from build123d import *

# Parameters (mm, degrees)
SKETCH_1_R          = 11
EXTRUDE_1_DEPTH     = 3.5
SKETCH_2_R          = 5
EXTRUDE_2_DEPTH     = 11.5
SKETCH_3_R          = 4
CUT_EXTRUDE_1_DEPTH = 22.610182785
SKETCH_4_R          = 1.75
CUT_EXTRUDE_2_DEPTH = 20.345542122


with BuildPart() as part:
    # 草图1 → 凸台-拉伸1 (new body)
    with BuildSketch(Plane(origin=(0, 0, 0), x_dir=(1, 0, 0), z_dir=(0, 1, 0))):
        with Locations(Location((0, 0, 0), (0, 0, 270))):
            Circle(SKETCH_1_R)
    extrude(amount=EXTRUDE_1_DEPTH)

    # 草图2 → 凸台-拉伸2 (add)
    with BuildSketch(Plane(origin=(0, 3.5, 0), x_dir=(1, 0, 0), z_dir=(0, 1, 0))):
        with Locations(Location((0, 0, 0), (0, 0, 270))):
            Circle(SKETCH_2_R)
    extrude(amount=EXTRUDE_2_DEPTH)

    # 草图3 → 切除-拉伸1 (cut, through all)
    with BuildSketch(Plane(origin=(0, 15, 0), x_dir=(1, 0, 0), z_dir=(0, 1, 0))):
        with Locations(Location((0, 0, 0), (0, 0, 270))):
            Circle(SKETCH_3_R)
    extrude(amount=-CUT_EXTRUDE_1_DEPTH, mode=Mode.SUBTRACT)

    # 草图4 → 切除-拉伸2 (cut, through all)
    with BuildSketch(Plane(origin=(0, 3.5, 0), x_dir=(1, 0, 0), z_dir=(0, 1, 0))):
        with Locations(Location((0, 8, 0), (0, 0, 270))):
            Circle(SKETCH_4_R)
        with Locations(Location((8, 0, 0), (0, 0, 270))):
            Circle(SKETCH_4_R)
        with Locations(Location((0, -8, 0), (0, 0, 270))):
            Circle(SKETCH_4_R)
        with Locations(Location((-8, 0, 0), (0, 0, 270))):
            Circle(SKETCH_4_R)
    extrude(amount=-CUT_EXTRUDE_2_DEPTH, mode=Mode.SUBTRACT)


solid = part.part
The model under review builds one solid part; all positions refer to its coordinate system, in mm. A direction names the side the tool comes from. Round coordinates to 2 decimals unless told otherwise and drop trailing zeros. Loops run counter-clockwise (first coordinate to the right, second up) from the corner with the lowest first, then second, coordinate; pieces in that order, holes last. Notation, with made-up numbers: (-12, 7.5) -> (43, 7.5) arc R35 ccw to (43, 43.5) -> close; hole circle Ø6 at (55, -35). An arc over 180 degrees is marked (long way). Return JSON: item names as keys, results as strings.
(1) Add section C-C on x = 7. Write out the cut boundary in (y, z), plus the area to 3 significant figures.
Solved:
{"outline": "(0, -8.49) -> (3.5, -8.49) -> (3.5, -1.44) -> (0, -1.44) -> close; (0, 1.44) -> (3.5, 1.44) -> (3.5, 8.49) -> (0, 8.49) -> close", "area": "49.3 mm2"}
(2) The part is to be moulded in two halves that separate along Z. For faces 3 (the cylindrical face through (-3.905, 7.605, -0.867)), 4 (the cylindrical face through (-10.74, 1.73, -2.38)), 5 (the cylindrical face through (0.526, 1.774, 9.669)), 6 (the flat face through (-5, 3.5, 2)), say which applies: released by +Z, released by -Z, zero draft, split by the parting line, or undercut.
Solved:
{"face 3": "undercut", "face 4": "split by the parting line", "face 5": "undercut", "face 6": "zero draft"}
(3) For faces 1 (the cylindrical face through (-4.88, 9.17, -1.08)), 2 (the cylindrical face through (-9.55, 1.77, 0.81)), list the 3-axis set-ups (+Z, -Z, +X, -X, +Y, -Y) from which the entire face can be reached by the end or side of a thin tool; tool diameter is ignored.
Solved:
{"face 1": "+Y", "face 2": "+Y, -Y"}
(4) Add section D-D on y = 10.5. Write out the cut boundary in (x, z), plus the area to 3 significant figures.
Solved:
{"outline": "circle Ø10 at (0, 0); hole circle Ø8 at (0, 0)", "area": "28.3 mm2"}
(5) For line 1 (X direction, y = 1.65, z = 0); line 2 (Y direction, x = 5.5, z = -0.5); line 3 (Z direction, x = 2, y = 3.75), list the stretches that pass through material, from the lowest coordinate up.
Solved:
{"line 1": "-11 to -9.75, -6.25 to -4, 4 to 6.25, 9.75 to 11", "line 2": "0 to 3.5", "line 3": "-4.58 to -3.46, 3.46 to 4.58"}
(6) Add section A-A on x = 0. Write out the cut boundary in (y, z), plus the area to 3 significant figures.
Solved:
{"outline": "(0, -11) -> (3.5, -11) -> (3.5, -9.75) -> (0, -9.75) -> close; (0, -6.25) -> (3.5, -6.25) -> (3.5, -5) -> (15, -5) -> (15, -4) -> (0, -4) -> close; (0, 4) -> (15, 4) -> (15, 5) -> (3.5, 5) -> (3.5, 6.25) -> (0, 6.25) -> close; (0, 9.75) -> (3.5, 9.75) -> (3.5, 11) -> (0, 11) -> close", "area": "47.5 mm2"}
(7) Add section B-B on z = -2.75. Write out the cut boundary in (x, y).
Solved:
{"outline": "(-10.65, 0) -> (-2.9, 0) -> (-2.9, 15) -> (-4.18, 15) -> (-4.18, 3.5) -> (-10.65, 3.5) -> close; (2.9, 0) -> (10.65, 0) -> (10.65, 3.5) -> (4.18, 3.5) -> (4.18, 15) -> (2.9, 15) -> close"}
(8) For pin 1 (1 mm diameter, centred on y = 8, z = -0.5, fed in from +X); pin 2 (8 mm diameter, centred on y = 5.5, z = -4, fed in from +X); pin 3 (3 mm diameter, centred on x = 8, z = 0, fed in from +Y); pin 4 (1 mm diameter, centred on y = 13, z = 3.5, fed in from -X), all flat-tipped, find the tip position at first contact; note any pin that passes through.
Solved:
{"pin 1": "x = 5", "pin 2": "x = 10.99", "pin 3": "through", "pin 4": "x = -4"}
